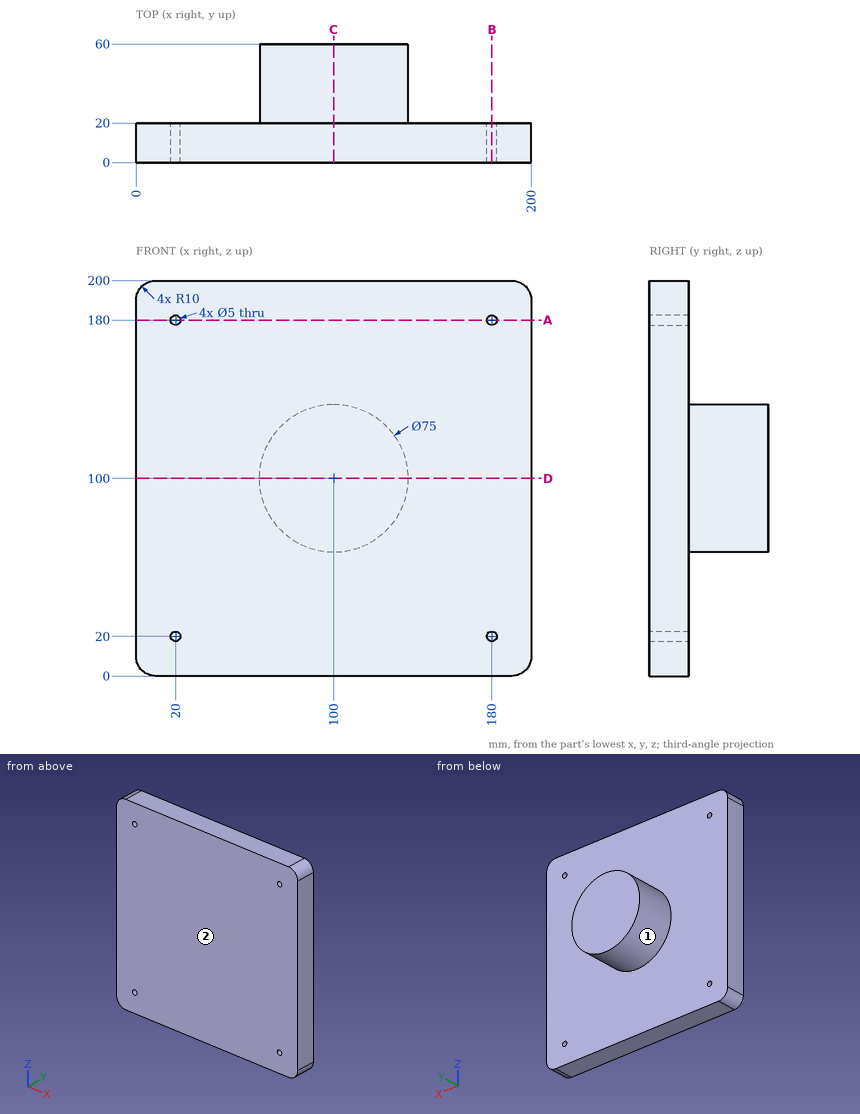
Drawing for the job (mm, zero at the part's lowest x, y, z). A direction names the side the tool comes from. Round coordinates to 2 decimals unless told otherwise and drop trailing zeros. Order: outer loops, then holes, each group sorted by start corner. A loop starts at its lowest first (then second) coordinate and runs counter-clockwise, first axis right, second up.
Item 1: Saw through at C-C on x = 100. Write the cut outline in (y, z), then the cut area to 3 significant figures.
Item 2: Tool access for the marked faces 1 and 2: list every direction of +Z, -Z, +X, -X, +Y, -Y with a clear straight run to the whole face (end or side of a thin tool).
Item 3: Saw through at B-B on x = 180. Write the cut outline in (y, z), then the cut area to 3 significant figures.
Item 4: Pin check, flat tips, straight feed: pin 1 (12 mm diameter, centred on x = 87.5, y = 53, fed in from -Z); pin 2 (12 mm diameter, centred on y = 47, z = 68, fed in from -X); pin 3 (6 mm diameter, centred on y = 23.5, z = 97.5, fed in from +X). Stop position of each tip, or through.
Item 5: Saw through at A-A on z = 180. Write the cut outline in (x, y).
Item 6: Saw through at D-D on z = 100. Write the cut outline in (x, y), then the cut area to 3 significant figures.
Item 7: Probe line 1 along X through (y, z) = (5.5, 180); line 2 along Y through (x, z) = (37, 70.5); line 3 along X through (y, z) = (34, 110). List the from-to ranges inside material, lowest first.
Reported:
1. outline: (0, 0) - (20, 0) - (20, 62.5) - (60, 62.5) - (60, 137.5) - (20, 137.5) - (20, 200) - (0, 200) - close
1. area: 7,000 mm2
2. face 1: +Y
2. face 2: +Z, -Z, +X, -X, -Y
3. outline: (0, 0) - (20, 0) - (20, 17.5) - (0, 17.5) - close; (0, 22.5) - (20, 22.5) - (20, 177.5) - (0, 177.5) - close; (0, 182.5) - (20, 182.5) - (20, 200) - (0, 200) - close
3. area: 3,800 mm2
4. pin 1: stops at z = 63.07
4. pin 2: stops at x = 72.98
4. pin 3: stops at x = 137.5
5. outline: (0, 0) - (17.5, 0) - (17.5, 20) - (0, 20) - close; (22.5, 0) - (177.5, 0) - (177.5, 20) - (22.5, 20) - close; (182.5, 0) - (200, 0) - (200, 20) - (182.5, 20) - close
6. outline: (0, 0) - (200, 0) - (200, 20) - (137.5, 20) - (137.5, 60) - (62.5, 60) - (62.5, 20) - (0, 20) - close
6. area: 7,000 mm2
7. line 1: x = 0 to 17.5, 22.5 to 177.5, 182.5 to 200
7. line 2: y = 0 to 20
7. line 3: x = 63.86 to 136.14
